CAD build for the part. Positions are in the model's coordinates, mm. Face numbers are marked on the shaded views. A direction names the side the tool comes from. Coordinates: 2 decimals unless noted, no trailing zeros. Order: outer loops, then holes, each group sorted by start corner. A loop starts at its lowest first (then second) coordinate and runs counter-clockwise, first axis right, second up. Notation, with made-up numbers: M 75.5,83.5 L 127.5,83.5 A21 ccw 127.5,99.5 Z; hole C 21.5,47 d2. An arc over 180 degrees is marked long. One line per item, written item: value.
Autodesk Inventor part; units mm, degrees
ref_plane "Work Plane1" through (-12, 0, 0) normal (1, 0, 0) x (0, 1, 0)
ref_plane "Work Plane2" through (-12, 0, 22) normal (0, 0, 1) x (1, 0, 0)
ref_plane "Work Plane3" through (-12, 0, 2) normal (0, 0, 1) x (1, 0, 0)
sketch "Sketch1" plane through (0, 0, 0) normal (0, 0, 1) x (1, 0, 0)
  line L0 (0, 0) -> (65, 0)
  circle A0 centre (0, 0) radius 12
  circle A1 centre (65, 0) radius 12
  line L1 (0, 12) -> (65, 12)
  line L2 (0, -12) -> (65, -12)
  dimension "d0" = 65
  dimension "d1" = 24
extrude "Extrusion1" add sketch "Sketch1" along normal blind 24
sketch "Sketch2" plane through (0, 0, 24) normal (0, 0, 1) x (1, 0, 0)
  circle A0 centre (0, 0) radius 6
  arc A1 (65, -12) -> (65, 12) centre (65, 0) ccw
  circle A2 centre (65, 0) radius 6
  line L0 (0, 6) -> (65, 6)
  line L1 (0, -6) -> (65, -6)
  dimension "d4" = 12
extrude "Extrusion2" cut sketch "Sketch2" against normal through all
sketch "Sketch3" plane through (0, 12, 0) normal (0, 1, 0) x (1, 0, 0)
  point P0 (0, 0)
  point P1 (32.5, -12)
hole "Hole1" at (32.5, 12, 12) direction (0, -1, 0) diameter 9 end through all
ref_plane "Work Plane1" through (-12, 0, 0) normal (1, 0, 0) x (0, 1, 0)
sketch "Sketch4" plane through (-12, 0, 0) normal (1, 0, 0) x (0, 1, 0)
  circle A0 centre (0, 12) radius 10
  point P0 (0, 0)
  dimension "d14" = 20
extrude "Extrusion3" add sketch "Sketch4" along normal blind 6
sketch "Sketch5" plane through (-12, 0, 0) normal (1, 0, 0) x (0, 1, 0)
  arc A0 (0, 22) -> (0, 2) centre (0, 12) ccw
  circle A1 centre (0, 12) radius 10
  point P0 (0, 0)
  point P1 (0, 2)
  dimension "d17" = 20
extrude "Extrusion4" add sketch "Sketch5" against normal blind 91
sketch "Sketch6" plane through (-103, 0, 12) normal (-1, 0, 0) x (0, 0, 1)
  circle A0 centre (0, 0) radius 8
  point P0 (-12, 0)
  dimension "d20" = 16
extrude "Extrusion5" add sketch "Sketch6" along normal blind 30
chamfer "Chamfer1" distance 3 angle 45 1 edges at (-133, 0, 4) measured on face at (-133, -1.0645, 14.108)
ref_plane "Work Plane2" through (-12, 0, 22) normal (0, 0, 1) x (1, 0, 0)
sketch "Sketch7" plane through (-12, 0, 22) normal (0, 0, 1) x (1, 0, 0)
  line L0 (-91, -10) -> (5.3668, -10)
  line L1 (-91, 10) -> (5.3668, 10)
  line L2 (-91, 10) -> (-91, -10)
  line L3 (-91, -10) -> (-71, -10)
  line L4 (-71, -10) -> (-71, 10)
  line L5 (-71, 10) -> (-91, 10)
  line L6 (-91, 10) -> (-91, -10)
  point P0 (12, 0)
  point P1 (-71, -10)
  dimension "d26" = 20
extrude "Extrusion6" cut sketch "Sketch7" against normal blind 2
ref_plane "Work Plane3" through (-12, 0, 2) normal (0, 0, 1) x (1, 0, 0)
sketch "Sketch8" plane through (-12, 0, 2) normal (0, 0, 1) x (1, 0, 0)
  line L0 (-91, -10) -> (5.3668, -10)
  line L1 (-91, 10) -> (-91, -10)
  line L2 (-91, 10) -> (5.3668, 10)
  line L3 (-91, -10) -> (-71, -10)
  line L4 (-71, -10) -> (-71, 10)
  line L5 (-71, 10) -> (-91, 10)
  line L6 (-91, 10) -> (-91, -10)
  point P0 (12, 0)
  point P1 (-91, 6)
  point P2 (-91, -6)
  point P3 (-71, -10)
  dimension "d29" = 20
extrude "Extrusion7" cut sketch "Sketch8" along normal blind 2
properties part number "hf2"
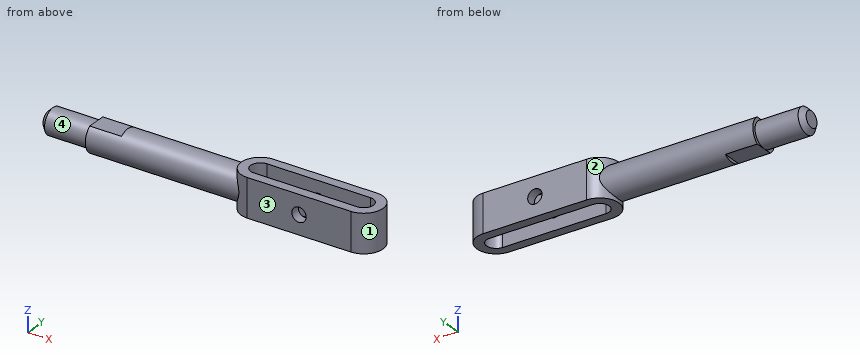
Q1. Pin check, flat tips, straight feed: pin 1 Ø5 at (x, z) = (-26.5, 14) entering from -Y; pin 2 Ø13 at (x, y) = (-90.5, -2.5) entering from +Z; pin 3 Ø8 at (x, y) = (-23.5, 8) entering from -Z. Stop position of each tip, or through.
Recorded:
pin 1: stops at y = -10
pin 2: stops at z = 20
pin 3: stops at z = 2.83
Q2. Which spindle directions (+Z, -Z, +X, -X, +Y, -Y) get a long thin tool onto all of the face, cutting with end or side? Do the marked faces 1 and 2. Say none if no direction does.
Recorded:
face 1: +Z, -Z, +X
face 2: -X
Q3. Drill centre lines: line 1 along X through (y, z) = (10.4, 12); line 2 along Y through (x, z) = (8.5, 1); line 3 along Z through (x, y) = (32.5, 9.2). Where is each one in solid material? Low to high.
Recorded:
line 1: x = -5.99 to 28, 37 to 70.99
line 2: y = -12 to -6, 6 to 12
line 3: z = 0 to 7.5, 16.5 to 24
Q4. Mould opens along Z. For the marked faces 3 and 4 say: released by +Z, released by -Z, zero draft, split by the parting line, or undercut.
Recorded:
face 3: zero draft
face 4: split by the parting line
Q5. Slice it at B-B (x = 32.5). List the corners of the cut face in (y, z).
Recorded:
outline: M -12,0 L -6,0 L -6,7.5 L -12,7.5 Z; M -12,16.5 L -6,16.5 L -6,24 L -12,24 Z; M 6,0 L 12,0 L 12,7.5 L 6,7.5 Z; M 6,16.5 L 12,16.5 L 12,24 L 6,24 Z
Q6. Slice it at A-A (x = 62). List the corners of the cut face in (y, z), plus the area to 3 significant figures.
Recorded:
outline: M -12,0 L -6,0 L -6,24 L -12,24 Z; M 6,0 L 12,0 L 12,24 L 6,24 Z
area: 288 mm^2
